Input: part model. Units: mm. Frame: model coordinates. Round coordinates to 2 decimals unless told otherwise and drop trailing zeros. Loops run counter-clockwise (first coordinate to the right, second up) from the corner with the lowest first, then second, coordinate; pieces in that order, holes last.
(1) Cut plane C-C, the plane x = 0.5. Output: boundary loops of the cut face in (y, z), and give its area (3 significant figures).
(2) Line query: line 1 (Z direction, x = -75.5, y = 0.8); line 2 (Z direction, x = -7, y = -0.8); line 3 (X direction, y = 1, z = -67). Output: solid intervals per line, ascending.
(3) Cut plane D-D, the plane z = 42. Output: boundary loops of the cut face in (x, y).
(4) Draft query along X for faces 1 (the face through (-89.15, -1.01, 89.91)), 2 (the face through (-1, 0, 1)), 3 (the face through (-52.385, -1.014, -42.324)), 4 (the face through (-1, -2, 1)). Return one class per face: released by +X, released by -X, zero draft, split by the parting line, or undercut.
(5) First-contact query: pin 1 Ø2 at (x, z) = (49.5, 71) entering from +Y; pin 2 Ø0.6 at (x, y) = (-1.5, 0.5) entering from -Z; pin 3 Ø0.6 at (y, z) = (1, -6) entering from +X. Flat tips, straight axial feed; report the tip coordinate or a pass-through.
(6) Cut plane A-A, the plane z = -46.46. Output: boundary loops of the cut face in (x, y).
(7) Cut plane B-B, the plane y = -1.15. Output: boundary loops of the cut face in (x, z), and give its area (3 significant figures).
from build123d import *

# Parameters (mm, degrees)
BOSS_EXTRUDE1_DEPTH = 2
SKETCH13_W          = 184
SKETCH13_H          = 185.84
SKETCH13_R          = 1.4
BOSS_EXTRUDE6_DEPTH = 2
FILLET3_R           = 10
CUT_EXTRUDE9_REACH  = 6
SKETCH14_R          = 6.12
SKETCH14_W          = 71.67
SKETCH14_H          = 24.82
SKETCH14_W_2        = 13.16
SKETCH14_H_2        = 20.24


with BuildPart() as part:
    # Sketch1 → Boss-Extrude1 (new body)
    with BuildSketch(Plane(origin=(0, 0, 0), x_dir=(1, 0, 0), z_dir=(0, 1, 0))):
        Polygon((-82.7, -90.62), (82.7, -90.62), (82.7, -83.62), (89.7, -83.62), (89.7, 83.62), (82.7, 83.62), (82.7, 90.62), (-82.7, 90.62), (-82.7, 83.62), (-89.7, 83.62), (-89.7, -83.62), (-82.7, -83.62), align=None)
        Polygon((-80.7, -88.62), (80.7, -88.62), (80.7, -81.62), (87.7, -81.62), (87.7, 81.62), (80.7, 81.62), (80.7, 88.62), (-80.7, 88.62), (-80.7, 81.62), (-87.7, 81.62), (-87.7, -81.62), (-80.7, -81.62), align=None, mode=Mode.SUBTRACT)
    extrude(amount=BOSS_EXTRUDE1_DEPTH)

    # Sketch13 → Boss-Extrude6 (add)
    with BuildSketch(Plane.XZ):
        Rectangle(SKETCH13_W, SKETCH13_H)
        with Locations((-86.5, -87.42)):
            Circle(SKETCH13_R, mode=Mode.SUBTRACT)
        with Locations((86.5, -87.42)):
            Circle(SKETCH13_R, mode=Mode.SUBTRACT)
        with Locations((86.5, 87.42)):
            Circle(SKETCH13_R, mode=Mode.SUBTRACT)
        with Locations((-86.5, 87.42)):
            Circle(SKETCH13_R, mode=Mode.SUBTRACT)
    extrude(amount=BOSS_EXTRUDE6_DEPTH)

    # Fillet3
    fillet3_edges = [part.edges().sort_by_distance(p)[0] for p in [
        (-92, -1, 92.92),
        (-92, -1, -92.92),
        (92, -1, -92.92),
        (92, -1, 92.92),
    ]]
    fillet(fillet3_edges, radius=FILLET3_R)

    # Sketch14 → Cut-Extrude9 (cut, up to next)
    with BuildSketch(Plane.XZ.offset(2), mode=Mode.PRIVATE) as cut_extrude9_sk1:
        with Locations((-47.874498459, -46.46)):
            Circle(SKETCH14_R)
    cut_extrude9_tool1 = extrude(cut_extrude9_sk1.sketch, amount=-CUT_EXTRUDE9_REACH, mode=Mode.PRIVATE) & part.part
    add(cut_extrude9_tool1.solids().sort_by_distance((-47.874498, -2, -46.46))[0], mode=Mode.SUBTRACT)
    # Sketch14 → Cut-Extrude9 (cut, up to next)
    with BuildSketch(Plane.XZ.offset(2), mode=Mode.PRIVATE) as cut_extrude9_sk2:
        with Locations((18.159498459, -46.46)):
            Rectangle(SKETCH14_W, SKETCH14_H)
    cut_extrude9_tool2 = extrude(cut_extrude9_sk2.sketch, amount=-CUT_EXTRUDE9_REACH, mode=Mode.PRIVATE) & part.part
    add(cut_extrude9_tool2.solids().sort_by_distance((18.159498, -2, -46.46))[0], mode=Mode.SUBTRACT)
    # Sketch14 → Cut-Extrude9 (cut, up to next)
    with BuildSketch(Plane.XZ.offset(2), mode=Mode.PRIVATE) as cut_extrude9_sk3:
        with Locations((56.12, 58.5)):
            Rectangle(SKETCH14_W_2, SKETCH14_H_2)
    cut_extrude9_tool3 = extrude(cut_extrude9_sk3.sketch, amount=-CUT_EXTRUDE9_REACH, mode=Mode.PRIVATE) & part.part
    add(cut_extrude9_tool3.solids().sort_by_distance((56.12, -2, 58.5))[0], mode=Mode.SUBTRACT)


solid = part.part
Reported:
1. outline: (-2, -92.92) - (0, -92.92) - (0, -90.62) - (2, -90.62) - (2, -88.62) - (0, -88.62) - (0, -58.87) - (-2, -58.87) - close; (-2, -34.05) - (0, -34.05) - (0, 88.62) - (2, 88.62) - (2, 90.62) - (0, 90.62) - (0, 92.92) - (-2, 92.92) - close
1. area: 330 mm2
2. line 1: z = -90.62 to -88.62, 88.62 to 90.62
2. line 2: z = -92.92 to -58.87, -34.05 to 92.92
2. line 3: x = -89.7 to -87.7, 87.7 to 89.7
3. outline: (-92, -2) - (92, -2) - (92, 0) - (89.7, 0) - (89.7, 2) - (87.7, 2) - (87.7, 0) - (-87.7, 0) - (-87.7, 2) - (-89.7, 2) - (-89.7, 0) - (-92, 0) - close
4. face 1: released by -X
4. face 2: undercut
4. face 3: undercut
4. face 4: zero draft
5. pin 1: stops at y = 0
5. pin 2: stops at z = -90.62
5. pin 3: stops at x = 89.7
6. outline: (-92, -2) - (-53.99, -2) - (-53.99, 0) - (-87.7, 0) - (-87.7, 2) - (-89.7, 2) - (-89.7, 0) - (-92, 0) - close; (-41.75, -2) - (-17.68, -2) - (-17.68, 0) - (-41.75, 0) - close; (53.99, -2) - (92, -2) - (92, 0) - (89.7, 0) - (89.7, 2) - (87.7, 2) - (87.7, 0) - (53.99, 0) - close
7. outline: (-92, -82.92) arc R10 ccw to (-82, -92.92) - (82, -92.92) arc R10 ccw to (92, -82.92) - (92, 82.92) arc R10 ccw to (82, 92.92) - (-82, 92.92) arc R10 ccw to (-92, 82.92) - close; hole circle Ø2.8 at (-86.5, -87.42); hole circle Ø2.8 at (-86.5, 87.42); hole circle Ø12.24 at (-47.87, -46.46); hole (-17.68, -58.87) - (53.99, -58.87) - (53.99, -34.05) - (-17.68, -34.05) - close; hole (49.54, 48.38) - (62.7, 48.38) - (62.7, 68.62) - (49.54, 68.62) - close; hole circle Ø2.8 at (86.5, -87.42); hole circle Ø2.8 at (86.5, 87.42)
7. area: 31,900 mm2
